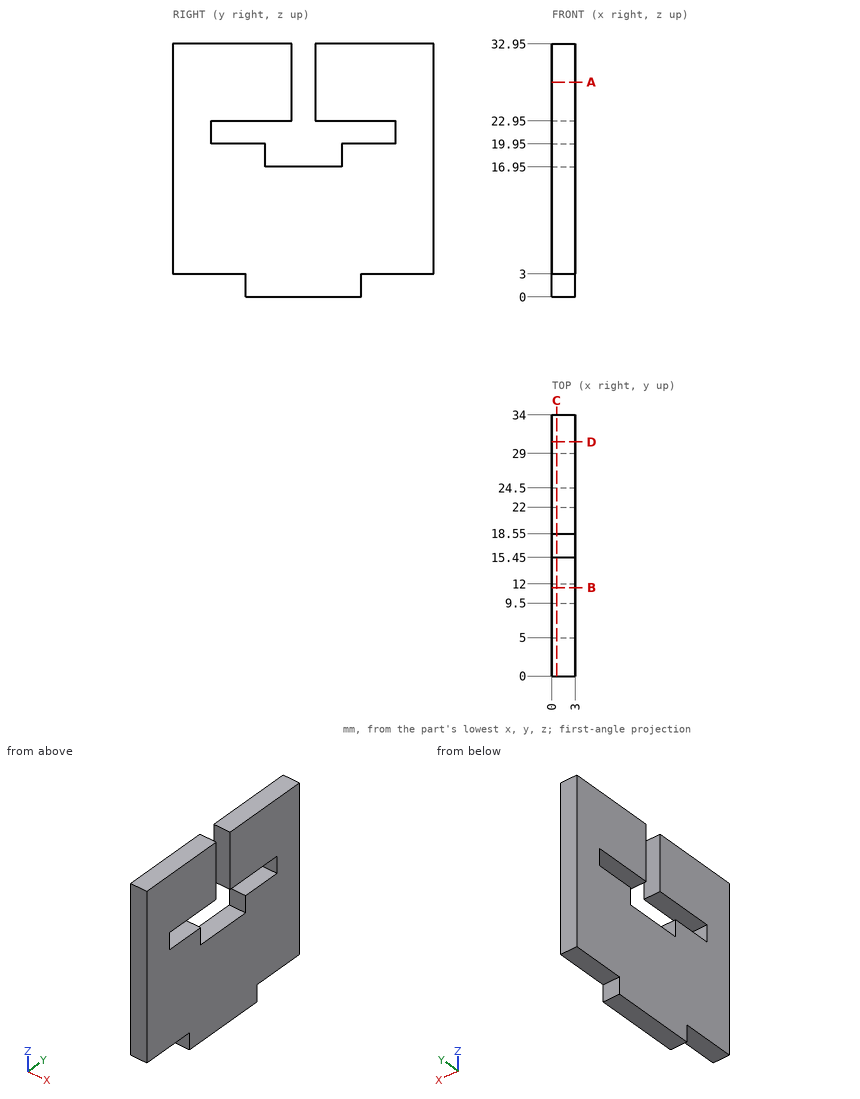
Input: dimensioned drawing with shaded views. Units: mm. Origin: part minimum x, y, z. Coordinates: 2 decimals unless noted, no trailing zeros. Write each loop counter-clockwise with the first axis right and the second up, starting at its lowest first coordinate (ties: lowest second). Pieces come first, ordered by that corner, then holes. Notation, with made-up numbers: M -22,12.25 L 23,12.25 A15 cw 23,39.25 Z; hole C 75.25,-33.5 d10. An arc over 180 degrees is marked long. Answer as CSV lines item,"result". Start each with the question number.
Q1. Cut plane C-C on x = 0.6. Return the cut outline in (y, z).
Q2. Cut plane D-D on y = 30.5. Return the cut outline in (x, z).
Q3. Cut plane B-B on y = 11.5. Return the cut outline in (x, z), then the cut area to 4 significant figures.
Q4. Cut plane A-A on z = 28. Return the cut outline in (x, y), then the cut area to 3 significant figures.
Q5. Line query: line 1 (Y direction, x = 0.65, z = 24); line 2 (Z direction, x = 2.6, y = 5.5); line 3 (Z direction, x = 0.9, y = 10.5). Output: solid intervals per line, ascending. Write a range as from..to.
Findings below:
1,outline,"M 0,3 L 9.5,3 L 9.5,0 L 24.5,0 L 24.5,3 L 34,3 L 34,32.95 L 18.55,32.95 L 18.55,22.95 L 29,22.95 L 29,19.95 L 22,19.95 L 22,16.95 L 12,16.95 L 12,19.95 L 5,19.95 L 5,22.95 L 15.45,22.95 L 15.45,32.95 L 0,32.95 Z"
2,outline,"M 0,3 L 3,3 L 3,32.95 L 0,32.95 Z"
3,outline,"M 0,0 L 3,0 L 3,19.95 L 0,19.95 Z; M 0,22.95 L 3,22.95 L 3,32.95 L 0,32.95 Z"
3,area,"89.85 mm2"
4,outline,"M 0,0 L 3,0 L 3,15.45 L 0,15.45 Z; M 0,18.55 L 3,18.55 L 3,34 L 0,34 Z"
4,area,"92.7 mm2"
5,line 1,"y = 0..15.45, 18.55..34"
5,line 2,"z = 3..19.95, 22.95..32.95"
5,line 3,"z = 0..19.95, 22.95..32.95"
